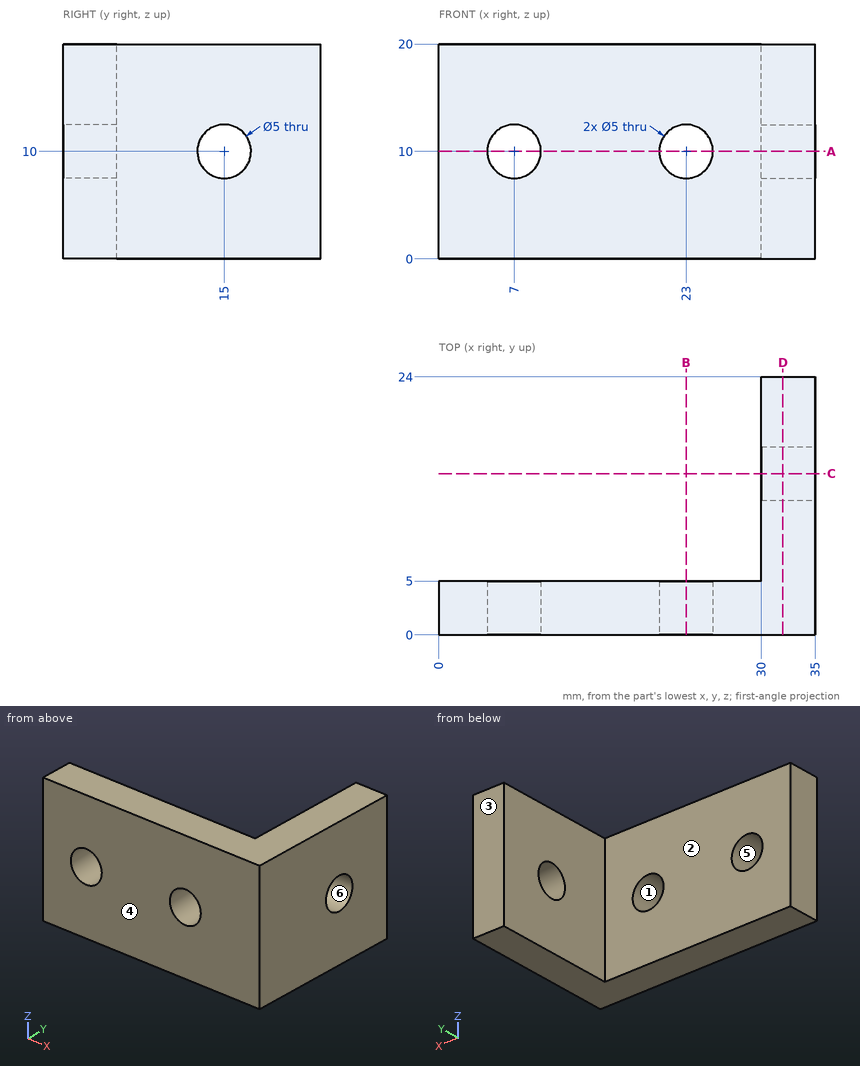
Job drawing, mm, ordinate dimensions from the low corner. One solid piece. A direction names the side the tool comes from. Coordinates: 2 decimals unless noted, no trailing zeros. Loops run counter-clockwise (first coordinate to the right, second up) from the corner with the lowest first, then second, coordinate; pieces in that order, holes last. Notation, with made-up numbers: (44, -4) - (60, -4) arc R17 cw to (60, 24) - close; hole circle Ø1 at (89.25, 77.25). An arc over 180 degrees is marked (long way). Answer as a JSON object with one key per item and string values. Group by question number.
(1) Flat gauge pins, fed straight in: pin 1 (8 mm diameter, centred on x = 7, z = 10, fed in from +Y); pin 2 (4 mm diameter, centred on x = 23, z = 10, fed in from +Y); pin 3 (2 mm diameter, centred on y = 18.5, z = 4.5, fed in from -X). Where does each tip first touch, or does it go through?
(2) Tool access for the marked faces 1 and 2: list every direction of +Z, -Z, +X, -X, +Y, -Y with a clear straight run to the whole face (end or side of a thin tool).
(3) Cut at B-B (x = 23). Give the cut face in (y, z), then the cut area to 3 significant figures.
(4) Cut at A-A (z = 10). Give the cut face in (x, y).
(5) Probe line 1 along X through (y, z) = (3.7, 10); line 2 along Z through (x, y) = (7, 2.85); line 3 along Y through (x, z) = (22.5, 4.25). List the from-to ranges inside material, lowest first.
(6) Cut at D-D (x = 32). Give the cut face in (y, z).
(7) Two-plate mould, pull along Y, no slides. Class the marked faces 3, 4, 5 and 6: released by +Y, released by -Y, zero draft, split by the parting line, or undercut.
(8) Cut at C-C (y = 15). Give the cut face in (x, z), then the cut area to 3 significant figures.
Geometry says:
{
 "1": {"pin 1": "stops at y = 5", "pin 2": "passes through", "pin 3": "stops at x = 30"},
 "2": {"face 1": "+Y, -Y", "face 2": "+Z, -Z, -X, +Y"},
 "3": {"outline": "(0, 0) - (5, 0) - (5, 7.5) - (0, 7.5) - close; (0, 12.5) - (5, 12.5) - (5, 20) - (0, 20) - close", "area": "75.0 mm^2"},
 "4": {"outline": "(0, 0) - (4.5, 0) - (4.5, 5) - (0, 5) - close; (9.5, 0) - (20.5, 0) - (20.5, 5) - (9.5, 5) - close; (25.5, 0) - (35, 0) - (35, 12.5) - (30, 12.5) - (30, 5) - (25.5, 5) - close; (30, 17.5) - (35, 17.5) - (35, 24) - (30, 24) - close"},
 "5": {"line 1": "x = 0 to 4.5, 9.5 to 20.5, 25.5 to 35", "line 2": "z = 0 to 7.5, 12.5 to 20", "line 3": "y = 0 to 5"},
 "6": {"outline": "(0, 0) - (24, 0) - (24, 20) - (0, 20) - close; hole circle Ø5 at (15, 10)"},
 "7": {"face 3": "released by +Y", "face 4": "released by -Y", "face 5": "zero draft", "face 6": "undercut"},
 "8": {"outline": "(30, 0) - (35, 0) - (35, 7.5) - (30, 7.5) - close; (30, 12.5) - (35, 12.5) - (35, 20) - (30, 20) - close", "area": "75.0 mm^2"}
}
